```python
from build123d import *
from build123d import SkipClean  # not in build123d's __all__

# Parameters (mm, degrees)
F1_DEPTH = 24
F2_DEPTH = 18
F3_DEPTH = 9.7
F4_DEPTH = 6
F5_DEPTH = 6
F6_R     = 1
F7_DEPTH = 4


with BuildPart() as f1:
    # F0 (on Top) → F1 (new body)
    with BuildSketch(Plane.XY):
        with BuildLine():
            ThreePointArc((0, -2.75), (1.9445436483, -1.9445436483), (2.75, 0))
            ThreePointArc((2.75, 0), (1.9445436483, 1.9445436483), (0, 2.75))
            Line((0, 2.75), (0, 1.12))
            Line((0, 1.12), (0, 0))
            Line((0, 0), (0, -1.13))
            Line((0, -1.13), (0, -2.75))
        make_face()
        with BuildLine():
            Line((0, 1.12), (0, 2.75))
            ThreePointArc((0, 2.75), (-0.5087835239, 2.7025246208), (-1, 2.5617376915))
            Line((-1, 2.5617376915), (-1, 1.12))
            Line((-1, 1.12), (0, 1.12))
        make_face()
        with BuildLine():
            ThreePointArc((-1, -2.5617376915), (-0.5087835239, -2.7025246208), (0, -2.75))
            Line((0, -2.75), (0, -1.13))
            Line((0, -1.13), (-1, -1.13))
            Line((-1, -1.13), (-1, -2.5617376915))
        make_face()
        with BuildLine():
            Line((-1, 1.12), (-1, 2.5617376915))
            ThreePointArc((-1, 2.5617376915), (-1.8980182962, 1.9899815445), (-2.5115931199, 1.12))
            Line((-2.5115931199, 1.12), (-1, 1.12))
        make_face()
        Polygon((0, 0), (0, 1.12), (-1, 1.12), (-1, -1.13), (0, -1.13), align=None)
        with BuildLine():
            ThreePointArc((-2.5071098899, -1.13), (-1.8940494052, -1.9937594767), (-1, -2.5617376915))
            Line((-1, -2.5617376915), (-1, -1.13))
            Line((-1, -1.13), (-2.5071098899, -1.13))
        make_face()
        with BuildLine():
            Line((-1, 1.12), (-2.5115931199, 1.12))
            ThreePointArc((-2.5115931199, 1.12), (-2.7499945409, -0.0054794925), (-2.5071098899, -1.13))
            Line((-2.5071098899, -1.13), (-1, -1.13))
            Line((-1, -1.13), (-1, 1.12))
        make_face()
    extrude(amount=F1_DEPTH)

    # F0 (on Top) → F2 (cut)
    with BuildSketch(Plane.XY):
        with BuildLine():
            Line((0, 1.12), (0, 2.75))
            ThreePointArc((0, 2.75), (-0.5087835239, 2.7025246208), (-1, 2.5617376915))
            Line((-1, 2.5617376915), (-1, 1.12))
            Line((-1, 1.12), (0, 1.12))
        make_face()
        with BuildLine():
            ThreePointArc((-1, -2.5617376915), (-0.5087835239, -2.7025246208), (0, -2.75))
            Line((0, -2.75), (0, -1.13))
            Line((0, -1.13), (-1, -1.13))
            Line((-1, -1.13), (-1, -2.5617376915))
        make_face()
        with BuildLine():
            Line((-1, 1.12), (-1, 2.5617376915))
            ThreePointArc((-1, 2.5617376915), (-1.8980182962, 1.9899815445), (-2.5115931199, 1.12))
            Line((-2.5115931199, 1.12), (-1, 1.12))
        make_face()
        Polygon((0, 0), (0, 1.12), (-1, 1.12), (-1, -1.13), (0, -1.13), align=None)
        with BuildLine():
            ThreePointArc((-2.5071098899, -1.13), (-1.8940494052, -1.9937594767), (-1, -2.5617376915))
            Line((-1, -2.5617376915), (-1, -1.13))
            Line((-1, -1.13), (-2.5071098899, -1.13))
        make_face()
        with BuildLine():
            Line((-1, 1.12), (-2.5115931199, 1.12))
            ThreePointArc((-2.5115931199, 1.12), (-2.7499945409, -0.0054794925), (-2.5071098899, -1.13))
            Line((-2.5071098899, -1.13), (-1, -1.13))
            Line((-1, -1.13), (-1, 1.12))
        make_face()
    extrude(amount=F2_DEPTH, mode=Mode.SUBTRACT)

    # F0 (on Top) → F3 (join)
    with BuildSketch(Plane.XY):
        with BuildLine():
            Line((0, 1.12), (0, 2.75))
            ThreePointArc((0, 2.75), (-0.5087835239, 2.7025246208), (-1, 2.5617376915))
            Line((-1, 2.5617376915), (-1, 1.12))
            Line((-1, 1.12), (0, 1.12))
        make_face()
        with BuildLine():
            ThreePointArc((-1, -2.5617376915), (-0.5087835239, -2.7025246208), (0, -2.75))
            Line((0, -2.75), (0, -1.13))
            Line((0, -1.13), (-1, -1.13))
            Line((-1, -1.13), (-1, -2.5617376915))
        make_face()
        Polygon((0, 0), (0, 1.12), (-1, 1.12), (-1, -1.13), (0, -1.13), align=None)
    extrude(amount=F3_DEPTH)

    # F0 (on Top) → F4 (join)
    with BuildSketch(Plane.XY):
        with BuildLine():
            Line((-1, 1.12), (-1, 2.5617376915))
            ThreePointArc((-1, 2.5617376915), (-1.8980182962, 1.9899815445), (-2.5115931199, 1.12))
            Line((-2.5115931199, 1.12), (-1, 1.12))
        make_face()
        with BuildLine():
            ThreePointArc((-2.5071098899, -1.13), (-1.8940494052, -1.9937594767), (-1, -2.5617376915))
            Line((-1, -2.5617376915), (-1, -1.13))
            Line((-1, -1.13), (-2.5071098899, -1.13))
        make_face()
        with BuildLine():
            Line((-1, 1.12), (-2.5115931199, 1.12))
            ThreePointArc((-2.5115931199, 1.12), (-2.7499945409, -0.0054794925), (-2.5071098899, -1.13))
            Line((-2.5071098899, -1.13), (-1, -1.13))
            Line((-1, -1.13), (-1, 1.12))
        make_face()
    extrude(amount=F4_DEPTH)

    # F0 (on Top) → F5 (join)
    with BuildSketch(Plane.XY):
        with BuildLine():
            ThreePointArc((-2.5071098899, -1.13), (-2.7499945409, -0.0054794925), (-2.5115931199, 1.12))
            Line((-2.5115931199, 1.12), (-6.75, 1.12))
            Line((-6.75, 1.12), (-6.75, -1.13))
            Line((-6.75, -1.13), (-2.5071098899, -1.13))
        make_face()
    extrude(amount=F5_DEPTH)

    # F6
    f6_edges = [f1.edges().sort_by_distance(p)[0] for p in [
        (-6.75, 1.12, 3),
        (-6.75, -1.13, 3),
    ]]
    fillet(f6_edges, radius=F6_R)

    # F0 (on Top) → F7 (cut)
    with BuildSketch(Plane.XY):
        with BuildLine():
            ThreePointArc((-2.5071098899, -1.13), (-2.7499945409, -0.0054794925), (-2.5115931199, 1.12))
            Line((-2.5115931199, 1.12), (-6.75, 1.12))
            Line((-6.75, 1.12), (-6.75, -1.13))
            Line((-6.75, -1.13), (-2.5071098899, -1.13))
        make_face()
    with SkipClean():  # cleaning this boolean's faces spoils the solid; the shape is the same uncleaned
        extrude(amount=F7_DEPTH, mode=Mode.SUBTRACT)


solid = f1.part
```
Geometry check sheet. Reference: the model listing, model coordinates, mm. A direction names the side the tool comes from. Give positions to 0.01 mm unless a question says otherwise; leave off trailing zeros. Loops run counter-clockwise (first coordinate to the right, second up) from the corner with the lowest first, then second, coordinate; pieces in that order, holes last. Notation, with made-up numbers: (22.5, -23.75) - (56.5, -23.75) arc R30 cw to (56.5, -1.75) - close; hole circle Ø11 at (50.25, 47). An arc over 180 degrees is marked (long way). Use CSV: the item, a comma, the result in double quotes. Start each with the question number.
Q1. Release check for a two-part mould opening along Z. For faces 1 (the face through (0, 0, 24)), 2 (the face through (0, 0, 14)), 3 (the face through (-3, 0, 6)), 4 (the face through (0, 0, 0)) record: +Z half, -Z half, draft (parallel to the pull), parting line (faces both ways), or undercut.
Q2. Section check D-D, the plane z = 22. Record the cut outline in (x, y), and give its area (3 significant figures).
Q3. Section check A-A, the plane y = -2.2. Record the cut outline in (x, z).
Q4. Scan lines: probe 1 along Z at (x, y) = (-5.25, -0.25); probe 2 along Z at (x, y) = (-0.5, -0.15); probe 3 along Z at (x, y) = (-1.5, -0.5). Record each from-to range of solid material in increasing order. Write a range as from..to.
Q5. Section check B-B, the plane z = 4.25. Record the cut outline in (x, y), and give its area (3 significant figures).
Q6. Go/stop test with flat-tipped pins: pin 1 Ø3 at (y, z) = (0.5, 12) entering from -X; pin 2 Ø1.6 at (x, z) = (-4, 5) entering from -Y; pin 3 Ø2 at (x, z) = (-4, 5) entering from +Y; pin 4 Ø3 at (x, z) = (-5.5, 20) entering from +Y. Record where each tip stops, or that it passes through.
Q7. Section check C-C, the plane x = -5.5. Record the cut outline in (y, z).
Q8. Access from +Z, -Z, +X, -X, +Y, -Y to the whole of each face (thin tool, end or side, straight path). Record for faces 5 (the face through (-4, -1.13, 5)), 6 (the face through (-4, 1.12, 5)), 7 (the face through (-1, 0, 8)).
Findings below:
1,face 1,"+Z half"
1,face 2,"undercut"
1,face 3,"undercut"
1,face 4,"-Z half"
2,outline,"circle Ø5.5 at (0, 0)"
2,area,"23.8 mm^2"
3,outline,"(-1.65, 0) - (1.65, 0) - (1.65, 24) - (-1.65, 24) - (-1.65, 18) - (0, 18) - (0, 9.7) - (-1, 9.7) - (-1, 6) - (-1.65, 6) - close"
4,probe 1,"z = 4..6"
4,probe 2,"z = 0..9.7, 18..24"
4,probe 3,"z = 0..6, 18..24"
5,outline,"(-6.75, -0.13) arc R1 ccw to (-5.75, -1.13) - (-2.51, -1.13) arc R2.75 ccw (long way) to (-2.51, 1.12) - (-5.75, 1.12) arc R1 ccw to (-6.75, 0.12) - close"
5,area,"32.5 mm^2"
6,pin 1,"stops at x = 0"
6,pin 2,"stops at y = -1.13"
6,pin 3,"stops at y = 1.12"
6,pin 4,"passes through"
7,outline,"(-1.13, 4) - (1.12, 4) - (1.12, 6) - (-1.13, 6) - close"
8,face 5,"+Z, -Z, -X, -Y"
8,face 6,"+Z, -Z, -X, +Y"
8,face 7,"-X, +Y, -Y"
